from build123d import *

# Parameters (mm, degrees)
BOSS_EXTRU_1_DEPTH = 2.2
BOSS_EXTRU_2_DEPTH = 6.1
CHANFREIN1_SIZE    = 1


with BuildPart() as part:
    # Esquisse1 → Boss.-Extru.1 (new body)
    with BuildSketch(Plane(origin=(0, 0, 0), x_dir=(1, 0, 0), z_dir=(0, 1, 0))):
        with BuildLine():
            Line((-6.1, 6.1), (6.1, 6.1))
            ThreePointArc((6.1, 6.1), (12.2, 0), (6.1, -6.1))
            Line((6.1, -6.1), (-6.1, -6.1))
            ThreePointArc((-6.1, -6.1), (-12.2, 0), (-6.1, 6.1))
        make_face()
    extrude(amount=BOSS_EXTRU_1_DEPTH)

    # Esquisse2 → Boss.-Extru.2 (add, symmetric)
    with BuildSketch(Plane.XY):
        Polygon((-2.1, 0), (-2.1, -2), (-1.7, -2.32091043), (-2.1, -3.5), (-3.3, -3.5), (-3.3, 0), align=None)
        Polygon((2.1, -3.5), (3.3, -3.5), (3.3, 0), (2.1, 0), (2.1, -2), (1.7, -2.32091043), align=None)
    extrude(amount=BOSS_EXTRU_2_DEPTH, both=True)

    # Chanfrein1
    chanfrein1_edges = [part.edges().sort_by_distance(p)[0] for p in [
        (-3.3, 0, 0),
        (3.3, 0, 0),
    ]]
    chamfer(chanfrein1_edges, length=CHANFREIN1_SIZE)


solid = part.part
The model under review builds one solid part; all positions refer to its coordinate system, in mm. A direction names the side the tool comes from. Round coordinates to 2 decimals unless told otherwise and drop trailing zeros. Loops run counter-clockwise (first coordinate to the right, second up) from the corner with the lowest first, then second, coordinate; pieces in that order, holes last. Notation, with made-up numbers: (14.25, 76) -> (21.25, 76) arc R16 ccw to (21.25, 95) -> close; hole circle Ø11 at (82.5, 34). An arc over 180 degrees is marked (long way). Return JSON: item names as keys, results as strings.
(1) For faces 4 (the flat face through (-3.3, -2, 0)), 5 (the flat face through (3.3, -2, 0)), 6 (the flat face through (-2.1, -1, 0)), list the 3-axis set-ups (+Z, -Z, +X, -X, +Y, -Y) from which the entire face can be reached by the end or side of a thin tool; tool diameter is ignored.
Solved:
{"face 4": "+Z, -Z, -X, -Y", "face 5": "+Z, -Z, +X, -Y", "face 6": "+Z, -Z"}
(2) Add section D-D on x = -0.75. Write out the cut boundary in (y, z), plus the area to 3 significant figures.
Solved:
{"outline": "(0, -6.1) -> (2.2, -6.1) -> (2.2, 6.1) -> (0, 6.1) -> close", "area": "26.8 mm2"}
(3) Add section B-B on z = 0. Write out the cut boundary in (x, y).
Solved:
{"outline": "(-12.2, 0) -> (-4.3, 0) -> (-3.3, -1) -> (-3.3, -3.5) -> (-2.1, -3.5) -> (-1.7, -2.32) -> (-2.1, -2) -> (-2.1, 0) -> (2.1, 0) -> (2.1, -2) -> (1.7, -2.32) -> (2.1, -3.5) -> (3.3, -3.5) -> (3.3, -1) -> (4.3, 0) -> (12.2, 0) -> (12.2, 2.2) -> (-12.2, 2.2) -> close"}
(4) Add section C-C on y = -0.35. Write out the cut boundary in (x, z), plus the area to 3 significant figures.
Solved:
{"outline": "(-3.95, -6.1) -> (-2.1, -6.1) -> (-2.1, 6.1) -> (-3.95, 6.1) -> close; (2.1, -6.1) -> (3.95, -6.1) -> (3.95, 6.1) -> (2.1, 6.1) -> close", "area": "45.1 mm2"}
(5) For line 1 (X direction, y = -1.25, z = -1.75); line 2 (Y direction, x = 8.75, z = -2.5); line 3 (X direction, y = -2.5, z = 2), list the stretches that pass through material, from the lowest coordinate up.
Solved:
{"line 1": "-3.3 to -2.1, 2.1 to 3.3", "line 2": "0 to 2.2", "line 3": "-3.3 to -1.76, 1.76 to 3.3"}
(6) The part is to be moulded in two halves that separate along X. For faces 1 (the cylindrical face through (12.2, 1.1, -0.1)), 2 (the flat face through (-3.8, -0.5, -0.1)), 3 (the flat face through (1.897, -2.902, 0.085)), say which applies: released by +X, released by -X, zero draft, split by the parting line, or undercut.
Solved:
{"face 1": "released by +X", "face 2": "released by -X", "face 3": "undercut"}
(7) Add section A-A on y = -1.5. Write out the cut boundary in (x, z).
Solved:
{"outline": "(-3.3, -6.1) -> (-2.1, -6.1) -> (-2.1, 6.1) -> (-3.3, 6.1) -> close; (2.1, -6.1) -> (3.3, -6.1) -> (3.3, 6.1) -> (2.1, 6.1) -> close"}
(8) For pin 1 (1.6 mm diameter, centred on y = -1, z = -2, fed in from -X); pin 2 (1.2 mm diameter, centred on y = -2.5, z = 2.5, fed in from +X); pin 3 (2 mm diameter, centred on y = -0.5, z = -3, fed in from +X); pin 4 (1.5 mm diameter, centred on x = 9, y = -1.5, fed in from +Z), all flat-tipped, find the tip position at first contact; note any pin that passes through.
Solved:
{"pin 1": "x = -4.1", "pin 2": "x = 3.3", "pin 3": "x = 11.81", "pin 4": "through"}
